CAD build for the part. Positions are in the model's coordinates, mm. A direction names the side the tool comes from. Coordinates: 2 decimals unless noted, no trailing zeros. Loops run counter-clockwise (first coordinate to the right, second up) from the corner with the lowest first, then second, coordinate; pieces in that order, holes last. Notation, with made-up numbers: (-37, 71) -> (-16, 71) arc R32 cw to (-16, 107) -> close; hole circle Ø11 at (18.25, 17). An arc over 180 degrees is marked (long way). Write each question's results on one line, items separated by ' | '.
from build123d import *

# Parameters (mm, degrees)
BLANKSKE_W        = 66
BLANKSKE_H        = 6.7
BLANK_DEPTH       = 3.4
TOOTHCUTSIM_DEPTH = 67.426274922
TEETHCUTS_COUNT   = 22
TEETHCUTS_PITCH   = 3.14159265
NOTCH_SKETCH_W    = 5.3
NOTCH_SKETCH_H    = 1.75
NOTCH_DEPTH       = 67.426274922


with BuildPart() as part:
    # BlankSke → Blank (new body)
    with BuildSketch(Plane.XY):
        with Locations((33, 3.35)):
            Rectangle(BLANKSKE_W, BLANKSKE_H)
    extrude(amount=-BLANK_DEPTH)

    # TooCutSkeSim → ToothCutSim (cut, through all)
    with BuildSketch(Plane.XY):
        Polygon((0.44443537, 4.45), (-0.44443537, 4.45), (-1.272613241, 6.7254), (1.272613241, 6.7254), align=None)
    toothcutsim = extrude(amount=-TOOTHCUTSIM_DEPTH, mode=Mode.SUBTRACT)

    # TeethCuts: ToothCutSim ×22
    with Locations(*[(i * TEETHCUTS_PITCH, 0, 0) for i in range(1, TEETHCUTS_COUNT)]):
        add(toothcutsim, mode=Mode.SUBTRACT)

    # notch-sketch → notch (cut, through all)
    with BuildSketch(Plane.XY):
        with Locations((6.65, 0.875)):
            Rectangle(NOTCH_SKETCH_W, NOTCH_SKETCH_H)
    extrude(amount=-NOTCH_DEPTH, mode=Mode.SUBTRACT)


solid = part.part
1) Two-plate mould, pull along X, no slides. Class faces 1 (the flat face through (65.125, 5.559, -1.676)), 2 (the flat face through (63.69, 5.59, -1.68)), 3 (the flat face through (33, 3, -3.4)): pulls with the +X half, pulls with the -X half, needs draft (parallel to the pull), parting line crosses it, or undercut.
Outcome:
face 1: pulls with the +X half | face 2: undercut | face 3: needs draft
2) Drill centre lines: L1, parallel to X at y = 0.5, z = -2.85; L2, parallel to Y at x = 16, z = -2.25. Where is each one in solid material? Low to high. Write a range as from..to.
Outcome:
L1: x = 0..4, 9.3..66 | L2: y = 0..4.45
3) Slice it at A-A (y = 0.75). Write the cut outline in (x, z), then the cut area to 3 significant figures.
Outcome:
outline: (0, -3.4) -> (4, -3.4) -> (4, 0) -> (0, 0) -> close; (9.3, -3.4) -> (66, -3.4) -> (66, 0) -> (9.3, 0) -> close | area: 206 mm^2
4) Pin check, flat tip, straight feed: pin 1 (1.7 mm diameter, centred on x = 7.5, z = -2, fed in from -Y). Stop position of the tip, or through.
Outcome:
pin 1: stops at y = 1.75
5) Slice it at B-B (y = 6). Count the separate pieces of the cut face and the enclosed holes in it, then the cut area to 3 significant figures.
Outcome:
separate pieces: 21 | enclosed holes: 0 | area: 80.3 mm^2
6) Which spindle directions (+Z, -Z, +X, -X, +Y, -Y) get a long thin tool onto all of the face, cutting with end or side? Do faces 4 (the flat face through (37, 0, -2)), 5 (the flat face through (7, 1.75, -2)), 6 (the flat face through (49.417, 5.559, -1.676)). Say none if no direction does.
Outcome:
face 4: +Z, -Z, +X, -X, -Y | face 5: +Z, -Z, -Y | face 6: +Z, -Z, +Y
